Design review of the part built by this model. Coordinates are the model's own, in mm. Coordinates: 2 decimals unless noted, no trailing zeros. Loops run counter-clockwise (first coordinate to the right, second up) from the corner with the lowest first, then second, coordinate; pieces in that order, holes last. Notation, with made-up numbers: (-27.5, 3) -> (-13.5, 3) arc R16 ccw to (-13.5, 17) -> close; hole circle Ø9 at (-12, 73). An arc over 180 degrees is marked (long way). Answer in a Markdown table with one row per item.
Autodesk Inventor part; units mm, degrees
ref_plane "YZ Plane" through (0, 0, 0) normal (1, 0, 0) x (0, 1, 0)
ref_plane "XZ Plane" through (0, 0, 0) normal (0, 1, 0) x (-1, 0, 0)
ref_plane "XY Plane" through (0, 0, 0) normal (0, 0, 1) x (1, 0, 0)
sketch "Sketch1" plane through (0, 0, 0) normal (0, 0, 1) x (1, 0, 0)
  line L0 (0, 3.75) -> (2, 3.75)
  line L1 (2, 3.75) -> (2, -4)
  line L2 (2, -4) -> (0, -4)
  line L3 (0, -4) -> (0, 3.75) construction
  line L4 (0, -4) -> (-5, -4)
  line L5 (-5, -4) -> (-5, -1)
  line L6 (-5, -1) -> (0, -1)
  line L7 (0, 3.75) -> (-1, 3.75)
  line L8 (-1, 3.75) -> (-1, 0.75)
  line L9 (-1, 0.75) -> (0, 0.75)
  line L10 (0, 0.75) -> (0, 3.75) construction
  line L11 (0, 0.75) -> (0, -1)
  point P0 (0, 0)
  point P1 (0, -0.125)
  point P2 (1, 3.75)
  dimension "d0" = 4
  dimension "d1" = 2
  dimension "d5" = 5
  dimension "d6" = 1.75
  dimension "d7" = 3
  dimension "d11" = 3
  dimension "d12" = 3
extrude "Extrusion1" add sketch "Sketch1" along normal blind 245.505
sketch "Sketch2" plane through (-1, 3.75, 245.505) normal (0, 1, 0) x (1, 0, 0)
  line L0 (3, 245.505) -> (3, 0) construction
  line L1 (3, 122.7525) -> (1, 122.7525) construction
  line L2 (1, 245.505) -> (1, 0) construction
  line L3 (3, 127.3525) -> (1, 127.3525)
  line L4 (1, 127.3525) -> (1, 118.1525) construction
  line L5 (1, 118.1525) -> (3, 118.1525) construction
  line L6 (3, 118.1525) -> (3, 127.3525)
  line L7 (3, 122.7525) -> (1, 122.7525) construction
  line L8 (3, 118.1525) -> (1, 118.1525)
  line L9 (1, 127.3525) -> (0, 127.3525)
  line L10 (0, 245.505) -> (0, 0)
  line L11 (0, 127.3525) -> (0, 118.1525)
  line L12 (0, 118.1525) -> (1, 118.1525)
  point P0 (0, 118.1525)
  dimension "d13" = 9.2
extrude "Extrusion2" cut sketch "Sketch2" against normal up to surface (3 mm away)
sketch "Sketch3" plane through (-1, 0.75, 0) normal (-1, 0, 0) x (0, 0, 1)
  line L0 (118.1525, 0) -> (118.1525, 3)
  line L1 (0, 3) -> (118.1525, 3)
  line L2 (0, 3) -> (0, 0)
  line L3 (0, 0) -> (118.1525, 0)
  line L4 (127.3525, 3) -> (127.3525, 0)
  line L5 (127.3525, 0) -> (245.505, 0)
  line L6 (245.505, 3) -> (245.505, 0)
  line L7 (127.3525, 3) -> (245.505, 3)
  point P0 (0, -0.75)
extrude "Extrusion3" cut sketch "Sketch3" against normal blind 0.9
chamfer "Chamfer1" distance 2.5 angle 45 1 edges at (-5, -4, 122.7525)
sketch "Sketch4" plane through (-0.1, 0.75, 0) normal (-1, 0, 0) x (0, 0, 1)
  line L0 (0, 3) -> (118.1525, 3)
  line L1 (0, 3) -> (2.45, 3)
  line L2 (2.45, 3) -> (2.45, 0.55)
  line L3 (2.45, 0.55) -> (0, 0.55)
  line L4 (0, 0.55) -> (0, 3)
  line L5 (127.3525, 3) -> (245.505, 3)
  line L6 (245.505, 3) -> (243.055, 3)
  line L7 (243.055, 3) -> (243.055, 0.55)
  line L8 (243.055, 0.55) -> (245.505, 0.55)
  line L9 (245.505, 0.55) -> (245.505, 3)
  line L10 (0, 3) -> (2.45, 3)
  line L11 (2.45, 3) -> (2.45, 0.55)
  line L12 (245.505, 3) -> (243.055, 3)
  line L13 (243.055, 3) -> (243.055, 0.55)
  point P0 (0, -0.75)
  dimension "d21" = 2.45
  dimension "d22" = 2.45
  dimension "d23" = 2.45
  dimension "d24" = 2.45
extrude "Extrusion4" add sketch "Sketch4" along normal blind 2.95
sketch "Sketch5" plane through (-0.1, 0.75, 0) normal (-1, 0, 0) x (0, 0, 1)
  line L0 (114.505, 2.85) -> (114.505, 0.85) construction
  line L1 (131, 0.85) -> (131, 2.85) construction
  line L2 (131, 2.85) -> (131, 3) construction
  line L3 (127.3525, 3) -> (243.055, 3) construction
  line L4 (114.505, 2.85) -> (114.505, 3) construction
  line L5 (114.505, 3) -> (118.1525, 3)
  line L6 (118.1525, 3) -> (118.1525, 1.05)
  line L7 (118.1525, 1.05) -> (114.505, 1.05)
  line L8 (114.505, 1.05) -> (114.505, 3)
  line L9 (131, 3) -> (127.3525, 3)
  line L10 (127.3525, 3) -> (127.3525, 1.05)
  line L11 (127.3525, 1.05) -> (131, 1.05)
  line L12 (131, 1.05) -> (131, 3)
  line L13 (2.45, 3) -> (118.1525, 3)
  line L14 (127.3525, 0) -> (127.3525, 3)
  line L15 (118.1525, 3) -> (118.1525, 0)
  point P0 (0, -0.75)
  dimension "d29" = 1.95
extrude "Extrusion5" add sketch "Sketch5" along normal blind 2.95
sketch "Sketch6" plane through (-0.1, 0.75, 0) normal (-1, 0, 0) x (0, 0, 1)
  line L0 (172.5025, 2.85) -> (172.5025, 0.85) construction
  line L1 (177.6025, 0.85) -> (177.6025, 2.85) construction
  line L2 (177.6025, 2.85) -> (177.6025, 3) construction
  line L3 (131, 3) -> (243.055, 3) construction
  line L4 (172.5025, 2.85) -> (172.5025, 3) construction
  line L5 (172.7025, 3) -> (177.4025, 3)
  line L6 (177.4025, 3) -> (177.4025, 1.05)
  line L7 (177.4025, 1.05) -> (172.7025, 1.05)
  line L8 (172.7025, 1.05) -> (172.7025, 3)
  point P0 (0, -0.75)
  dimension "d32" = 0.2
  dimension "d33" = 0.2
  dimension "d34" = 1.95
extrude "Extrusion6" add sketch "Sketch6" along normal blind 2.95
sketch "Sketch7" plane through (2, -4, 0) normal (1, 0, 0) x (0, 0, -1)
  line L0 (-7.6603, 5.3316) -> (-4.3041, 5.3316) construction
  line L1 (-4.3041, 5.3316) -> (-4.3041, 2.2816) construction
  line L2 (-4.3041, 2.2816) -> (-7.6603, 2.2816) construction
  line L3 (-7.6603, 2.2816) -> (-7.6603, 5.3316) construction
  line L4 (-7.3186, 5.3316) -> (-6.8833, 5.3316)
  line L5 (-6.8833, 5.3316) -> (-6.8833, 2.2816)
  line L6 (-6.8833, 2.2816) -> (-7.3186, 2.2816)
  line L7 (-7.3186, 2.2816) -> (-7.3186, 5.3316)
  line L8 (-6.1999, 5.3316) -> (-5.7645, 5.3316)
  line L9 (-5.7645, 5.3316) -> (-5.7645, 2.2816)
  line L10 (-5.7645, 2.2816) -> (-6.1999, 2.2816)
  line L11 (-6.1999, 2.2816) -> (-6.1999, 5.3316)
  line L12 (-5.0811, 5.3316) -> (-4.6458, 5.3316)
  line L13 (-4.6458, 5.3316) -> (-4.6458, 2.2816)
  line L14 (-4.6458, 2.2816) -> (-5.0811, 2.2816)
  line L15 (-5.0811, 2.2816) -> (-5.0811, 5.3316)
  point P0 (0, 4)
extrude "Extrusion7" cut sketch "Sketch7" against normal blind 1
properties part number "Top Case Rail" material "PET Plastic"
(1) Take a section at A-A on z = 49. Give the boundary of the cut face in (x, y).
Evaluation:
| item | result |
|---|---|
| outline | (-5, -1.5) -> (-2.5, -4) -> (2, -4) -> (2, 3.75) -> (-0.1, 3.75) -> (-0.1, 0.75) -> (0, 0.75) -> (0, -1) -> (-5, -1) -> close |
(2) To check wall thickness, follow probe 1 along Z at (x, y) = (1.75, 0) (1 decimal); probe 2 along Z at (x, y) = (0.75, 2) (1 decimal); probe 3 along Z at (x, y) = (-2.75, 1.75) (3 decimals). State the ranges of each line that lie inside material, in increasing order.
Evaluation:
| item | result |
|---|---|
| probe 1 | z = 0 to 4.6, 5.1 to 5.8, 6.2 to 6.9, 7.3 to 245.5 |
| probe 2 | z = 0 to 118.2, 127.4 to 245.5 |
| probe 3 | z = 0 to 2.45, 243.055 to 245.505 |
(3) For pin 1 (1.5 mm diameter, centred on x = -3.5, z = 128, fed in from -Y); pin 2 (1.6 mm diameter, centred on y = 2.5, z = 174, fed in from -X); pin 3 (1.5 mm diameter, centred on y = 3, z = 178.5, fed in from -X), all flat-tipped, find the tip position at first contact; note any pin that passes through.
Evaluation:
| item | result |
|---|---|
| pin 1 | stops at y = -3.75 |
| pin 2 | stops at x = -3.05 |
| pin 3 | stops at x = -0.1 |
